Geometry: final body of the model. Coordinates: model frame, mm. Coordinates: 2 decimals unless noted, no trailing zeros. Loops run counter-clockwise (first coordinate to the right, second up) from the corner with the lowest first, then second, coordinate; pieces in that order, holes last. Notation, with made-up numbers: (35, 14.25) - (59, 14.25) arc R14 cw to (59, 28.25) - close; hole circle Ø2 at (72.25, 36). An arc over 180 degrees is marked (long way). Put each result on its own line as item: value. Start each with the question number.
1) Section A-A on z = -85.09. Output: boundary loops of the cut face in (x, y), and give its area (3 significant figures).
2) Section B-B on y = -3.15. Count the separate pieces of the cut face and the enclosed holes in it, and give its area (3 significant figures).
3) Material intervals for line 1 along Z through (x, y) = (-34, -3.75); line 2 along X through (y, z) = (-1.3, 77.5); line 3 along X through (y, z) = (-0.6, -93.5), sorted ascending. Write a range as from..to.
4) Section C-C on x = 95. Output: boundary loops of the cut face in (y, z), and give its area (3 significant figures).
5) Contact query for flat-ended pins moving along their axis: pin 1 Ø2 at (y, z) = (-1.5, -88) entering from -X; pin 2 Ø1.5 at (y, z) = (-4, -49.5) entering from -X. Output: stop coordinate, or through.
6) Section D-D on z = 30. Output: boundary loops of the cut face in (x, y).
```python
from build123d import *

# Parameters (mm, degrees)
SKETCH1_R           = 117.475
BOSS_EXTRUDE1_DEPTH = 4.826
SKETCH5_R           = 1.778
CUT_EXTRUDE6_DEPTH  = 167.204817999
SKETCH6_R           = 1.778
CUT_EXTRUDE7_DEPTH  = 167.204817999
SKETCH7_R           = 1.778
CUT_EXTRUDE8_DEPTH  = 167.204817999
SKETCH8_R           = 12.7
CUT_EXTRUDE9_DEPTH  = 167.204817999
SKETCH9_R           = 1.905
CUT_EXTRUDE10_DEPTH = 167.204817999
CIRPATTERN1_COUNT   = 3
CIRPATTERN1_ANGLE   = 45
CIRPATTERN2_COUNT   = 3
CIRPATTERN2_ANGLE   = 45
SKETCH10_R          = 15.875
CUT_EXTRUDE11_DEPTH = 167.204817999


with BuildPart() as part:
    # Sketch1 → Boss-Extrude1 (new body)
    with BuildSketch(Plane(origin=(0, 0, 0), x_dir=(1, 0, 0), z_dir=(0, 1, 0))):
        with Locations(Location((0, 0, 0), (0, 0, 270))):
            Circle(SKETCH1_R)
    extrude(amount=-BOSS_EXTRUDE1_DEPTH)

    # Sketch5 → Cut-Extrude6 (cut, through all)
    with BuildSketch(Plane(origin=(0, 0, 0), x_dir=(1, 0, 0), z_dir=(0, 1, 0))):
        with Locations(Location((0, 0, 0), (0, 0, 270))):
            Circle(SKETCH5_R)
    extrude(amount=-CUT_EXTRUDE6_DEPTH, mode=Mode.SUBTRACT)

    # Sketch6 → Cut-Extrude7 (cut, through all)
    with BuildSketch(Plane(origin=(0, 0, 0), x_dir=(1, 0, 0), z_dir=(0, 1, 0))):
        with Locations(Location((0, 25.4, 0), (0, 0, 270))):
            Circle(SKETCH6_R)
        with Locations(Location((-12.7, 25.4, 0), (0, 0, 270))):
            Circle(SKETCH6_R)
        with Locations(Location((-25.4, 25.4, 0), (0, 0, 270))):
            Circle(SKETCH6_R)
        with Locations(Location((-38.1, 25.4, 0), (0, 0, 270))):
            Circle(SKETCH6_R)
        with Locations(Location((12.7, 25.4, 0), (0, 0, 270))):
            Circle(SKETCH6_R)
        with Locations(Location((25.4, 25.4, 0), (0, 0, 270))):
            Circle(SKETCH6_R)
        with Locations(Location((38.1, 25.4, 0), (0, 0, 270))):
            Circle(SKETCH6_R)
        with Locations(Location((-50.8, 25.4, 0), (0, 0, 270))):
            Circle(SKETCH6_R)
        with Locations(Location((50.8, 25.4, 0), (0, 0, 270))):
            Circle(SKETCH6_R)
        with Locations(Location((-63.5, 25.4, 0), (0, 0, 270))):
            Circle(SKETCH6_R)
        with Locations(Location((63.5, 25.4, 0), (0, 0, 270))):
            Circle(SKETCH6_R)
        with Locations(Location((0, 106.68, 0), (0, 0, 270))):
            Circle(SKETCH6_R)
        with Locations(Location((-12.7, 106.68, 0), (0, 0, 270))):
            Circle(SKETCH6_R)
        with Locations(Location((12.7, 106.68, 0), (0, 0, 270))):
            Circle(SKETCH6_R)
    extrude(amount=-CUT_EXTRUDE7_DEPTH, mode=Mode.SUBTRACT)

    # Sketch7 → Cut-Extrude8 (cut, through all)
    with BuildSketch(Plane(origin=(0, 0, 0), x_dir=(1, 0, 0), z_dir=(0, 1, 0))):
        with Locations(Location((0, 12.7, 0), (0, 0, 270))):
            Circle(SKETCH7_R)
        with Locations(Location((12.7, 0, 0), (0, 0, 270))):
            Circle(SKETCH7_R)
        with Locations(Location((0, -12.7, 0), (0, 0, 270))):
            Circle(SKETCH7_R)
        with Locations(Location((-12.7, 0, 0), (0, 0, 270))):
            Circle(SKETCH7_R)
        with Locations(Location((-8.980256121, 8.980256121, 0), (0, 0, 270))):
            Circle(SKETCH7_R)
        with Locations(Location((8.980256121, 8.980256121, 0), (0, 0, 270))):
            Circle(SKETCH7_R)
        with Locations(Location((8.980256121, -8.980256121, 0), (0, 0, 270))):
            Circle(SKETCH7_R)
        with Locations(Location((-8.980256121, -8.980256121, 0), (0, 0, 270))):
            Circle(SKETCH7_R)
    extrude(amount=-CUT_EXTRUDE8_DEPTH, mode=Mode.SUBTRACT)

    # Sketch8 → Cut-Extrude9 (cut, through all)
    with BuildSketch(Plane(origin=(0, 0, 0), x_dir=(1, 0, 0), z_dir=(0, 1, 0))):
        with Locations(Location((-35.921024484, -35.921024484, 0), (0, 0, 270))):
            Circle(SKETCH8_R)
    extrude(amount=-CUT_EXTRUDE9_DEPTH, mode=Mode.SUBTRACT)

    # Sketch9 → Cut-Extrude10 (cut, through all)
    with BuildSketch(Plane(origin=(0, 0, 0), x_dir=(1, 0, 0), z_dir=(0, 1, 0))):
        with Locations(Location((0, -82.55, 0), (0, 0, 270))):
            Circle(SKETCH9_R)
    cut_extrude10 = extrude(amount=-CUT_EXTRUDE10_DEPTH, mode=Mode.SUBTRACT)

    # CirPattern1: Cut-Extrude10 ×3 about axis
    cirpattern1_axis = Axis((0, 0, 0), (0, 1, 0))
    for i in range(1, CIRPATTERN1_COUNT):
        add(cut_extrude10.rotate(cirpattern1_axis, i * CIRPATTERN1_ANGLE / (CIRPATTERN1_COUNT - 1)), mode=Mode.SUBTRACT)

    # CirPattern2: Cut-Extrude10 ×3 about axis
    cirpattern2_axis = Axis((0, 0, 0), (0, -1, 0))
    for i in range(1, CIRPATTERN2_COUNT):
        add(cut_extrude10.rotate(cirpattern2_axis, i * CIRPATTERN2_ANGLE / (CIRPATTERN2_COUNT - 1)), mode=Mode.SUBTRACT)

    # Sketch10 → Cut-Extrude11 (cut, through all)
    with BuildSketch(Plane(origin=(0, 0, 0), x_dir=(1, 0, 0), z_dir=(0, 1, 0))):
        with Locations(Location((-19.812, 85.09, 0), (0, 0, 270))):
            Circle(SKETCH10_R)
    extrude(amount=-CUT_EXTRUDE11_DEPTH, mode=Mode.SUBTRACT)


solid = part.part
```
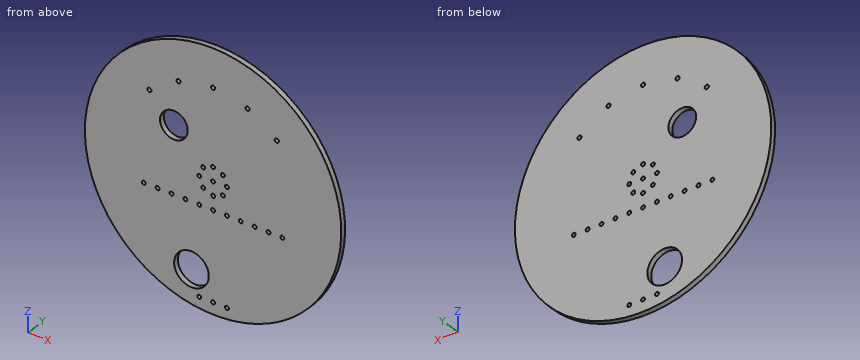
Answer block:
1. outline: (-80.99, -4.83) - (-35.69, -4.83) - (-35.69, 0) - (-80.99, 0) - close; (-3.94, -4.83) - (80.99, -4.83) - (80.99, 0) - (-3.94, 0) - close
1. area: 629 mm²
2. separate pieces: 1
2. enclosed holes: 30
2. area: 41,800 mm²
3. line 1: z = -112.45..-92.21, -77.97..23.37, 48.47..112.45
3. line 2: x = -88.28..-33.04, -30.14..30.14, 33.04..88.28
3. line 3: x = -71.12..-33.28, -6.35..71.12
4. outline: (-4.83, -69.1) - (0, -69.1) - (0, 69.1) - (-4.83, 69.1) - close
4. area: 667 mm²
5. pin 1: stops at x = -78.94
5. pin 2: stops at x = -106.88
6. outline: (-113.58, -4.83) - (-47.16, -4.83) - (-47.16, 0) - (-113.58, 0) - close; (-24.69, -4.83) - (113.58, -4.83) - (113.58, 0) - (-24.69, 0) - close
